Can you work these out from the model? Positions are in its coordinate system, mm. Face numbers are marked on the shaded views. A direction names the side the tool comes from. Round coordinates to 2 decimals unless told otherwise and drop trailing zeros. Loops run counter-clockwise (first coordinate to the right, second up) from the corner with the lowest first, then second, coordinate; pieces in that order, holes last. Notation, with made-up numbers: (-5, 70.25) - (50, 70.25) arc R24 cw to (50, 100.25) - close; hole circle Ø3 at (30.25, -13.5). An arc over 180 degrees is marked (long way). Answer as CSV lines item,"result".
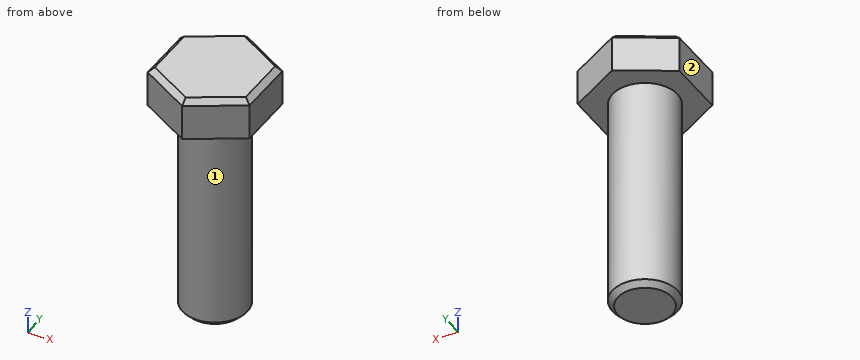
```python
from build123d import *

# Parameters (mm, degrees)
F0_R     = 6
F1_DEPTH = 20
F3_DEPTH = 7.55
F4_SIZE  = 1
F5_SIZE  = 1


with BuildPart() as f1:
    # F0 (on Top) → F1 (new body, symmetric)
    with BuildSketch(Plane.XY):
        Circle(F0_R)
    extrude(amount=F1_DEPTH, both=True)

    # F2 (on face) → F3 (join)
    with BuildSketch(Plane.XY.offset(20)):
        Polygon((0, 10.854185), (-9.4, 5.427093), (-9.4, -5.427093), (0, -10.854185), (9.4, -5.427093), (9.4, 5.427093), align=None)
    extrude(amount=F3_DEPTH)

    # F4
    f4_edges = [f1.edges().sort_by_distance(p)[0] for p in [
        (-6, 0, -20),
    ]]
    chamfer(f4_edges, length=F4_SIZE)

    # F5
    f5_edges = [f1.edges().sort_by_distance(p)[0] for p in [
        (4.7, 8.140639, 27.55),
        (-4.7, 8.140639, 27.55),
        (-9.4, 0, 27.55),
        (-4.7, -8.140639, 27.55),
        (4.7, -8.140639, 27.55),
        (9.4, 0, 27.55),
    ]]
    chamfer(f5_edges, length=F5_SIZE)


solid = f1.part
```
Q1. Imagine slicing it at B-B (y = -8.25). Write out the boundary of the cut face in (x, z), then the cut area to 3 significant figures.
Checks:
outline,"(-4.51, 20) - (4.51, 20) - (4.51, 26.55) - (2.51, 27.55) - (-2.51, 27.55) - (-4.51, 26.55) - close"
area,"66.1 mm²"
Q2. I'm going to push flat-ended pins straight in: pin 1 Ø3 at (y, z) = (6.5, 3.5) entering from -X; pin 2 Ø8 at (x, z) = (-3.5, 11.5) entering from -Y; pin 3 Ø4 at (y, z) = (2.5, -14) entering from -X; pin 4 Ø5 at (x, y) = (-6.5, 6) entering from +Z. Where does each tip first touch, or does it pass through?
Checks:
pin 1,"x = -3.32"
pin 2,"y = -6"
pin 3,"x = -5.98"
pin 4,"z = 27.55"
Q3. If I drill on line 1 along Z through (x, y) = (-1.25, -7.25); line 2 along Y through (x, z) = (2.5, 9.5); line 3 along Y through (x, z) = (-2, -7), over which ranges is the centre line in solid material (lowest first)? Write a range as [from, to].
Checks:
line 1,"[20, 27.55]"
line 2,"[-5.45, 5.45]"
line 3,"[-5.66, 5.66]"
Q4. On a 3-axis mill with a long thin cutter (end or side, diameter ignored), from which of +Z, -Z, +X, -X, +Y, -Y can I reach the whole of each face in a straight line? I mean the marked faces 1 and 2. Say none if no direction works.
Checks:
face 1,"-Z"
face 2,"+Z, -Z, -X, +Y, -Y"
Q5. Imagine slicing it at A-A (z = -6.5). Write out the boundary of the cut face in (x, y), then the cut area to 3 significant figures.
Checks:
outline,"circle Ø12 at (0, 0)"
area,"113 mm²"
